Model file for the job. Use its own axes, mm. A direction names the side the tool comes from. Give positions to 0.01 mm unless a question says otherwise; leave off trailing zeros. Loops run counter-clockwise (first coordinate to the right, second up) from the corner with the lowest first, then second, coordinate; pieces in that order, holes last. Notation, with made-up numbers: (46, 87.5) - (86, 87.5) arc R11 ccw to (86, 101.5) - close; hole circle Ø6 at (-24, -26.75). An arc over 180 degrees is marked (long way). Use a Markdown table: item, result.
from build123d import *

# Parameters (mm, degrees)
EXTRUDE_1_DEPTH               = 3
SKETCH_2_W                    = 40
SKETCH_2_H                    = 29
EXTRUDE_2_DEPTH               = 4.3
EXTRUDE_3_DEPTH               = 3
SKETCH_4_W                    = 35.7
SKETCH_4_H                    = 29
EXTRUDE_4_DEPTH               = 4.3
SKETCH_5_W                    = 36
SKETCH_5_H                    = 8
CUT_EXTRUDE_1_DEPTH           = 2
CUT_EXTRUDE_1_DRAFT           = -30
CUT_EXTRUDE_1_PROFILE_2_DEPTH = 2
CUT_EXTRUDE_1_PROFILE_2_DRAFT = -30
SKETCH_5_W_2                  = 23.5
SKETCH_5_H_2                  = 8.8
CUT_EXTRUDE_1_PROFILE_3_DEPTH = 2
CUT_EXTRUDE_1_PROFILE_3_DRAFT = -30
SKETCH_6_W                    = 36
SKETCH_6_H                    = 8
CUT_EXTRUDE_2_DEPTH           = 2
CUT_EXTRUDE_2_DRAFT           = -30
CUT_EXTRUDE_2_PROFILE_2_DEPTH = 2
CUT_EXTRUDE_2_PROFILE_2_DRAFT = -30
SKETCH_6_W_2                  = 23.5
SKETCH_6_H_2                  = 8.8
CUT_EXTRUDE_2_PROFILE_3_DEPTH = 2
CUT_EXTRUDE_2_PROFILE_3_DRAFT = -30
EXTRUDE_START                 = -3
EXTRUDE_5_DEPTH               = 6
EXTRUDE_6_DEPTH               = 3
FILLET_2_R                    = 0.2


# Read off the part's stored shape, not the designer's step: the extrude step
with BuildPart() as part:
    # Sketch 1 → Extrude 1 (new body)
    with BuildSketch(Plane(origin=(0, 0, 0), x_dir=(1, 0, 0), z_dir=(0, 1, 0))):
        Polygon((0, 0), (0, 40), (-8, 40), (-8, 32), (-32, 8), (-40, 8), (-40, 0), align=None)
    extrude(amount=EXTRUDE_1_DEPTH)

    # Sketch 2 → Extrude 2 (add)
    with BuildSketch(Plane(origin=(0, 0, 0), x_dir=(0, 0, -1), z_dir=(1, 0, 0))):
        with Locations((20, 17.5)):
            Rectangle(SKETCH_2_W, SKETCH_2_H)
        with BuildLine():
            Line((27, 13.1), (15, 13.1))
            ThreePointArc((15, 13.1), (10.6, 17.5), (15, 21.9))
            Line((15, 21.9), (27, 21.9))
            ThreePointArc((27, 21.9), (31.4, 17.5), (27, 13.1))
        make_face(mode=Mode.SUBTRACT)
    extrude(amount=-EXTRUDE_2_DEPTH)

    # Sketch 3 → Extrude 3 (add)
    with BuildSketch(Plane(origin=(0, 32, 0), x_dir=(1, 0, 0), z_dir=(0, 1, 0))):
        Polygon((-4.3, 40), (0, 40), (0, 0), (-4.3, 0), (-40, 0), (-40, 8), (-32, 8), (-8, 32), (-8, 40), align=None)
    extrude(amount=EXTRUDE_3_DEPTH)

    # Sketch 4 → Extrude 4 (add)
    with BuildSketch(Plane.XY):
        with Locations((-22.15, 17.5)):
            Rectangle(SKETCH_4_W, SKETCH_4_H)
        with BuildLine():
            Line((-27, 21.9), (-15, 21.9))
            ThreePointArc((-15, 21.9), (-10.6, 17.5), (-15, 13.1))
            Line((-15, 13.1), (-27, 13.1))
            ThreePointArc((-27, 13.1), (-31.4, 17.5), (-27, 21.9))
        make_face(mode=Mode.SUBTRACT)
    extrude(amount=-EXTRUDE_4_DEPTH)


with BuildPart() as cut_extrude_1_tool:
    # Sketch 5 → Cut-Extrude 1 (with draft: the straight prism first)
    with BuildSketch(Plane(origin=(0, 0, 0), x_dir=(0, 0, -1), z_dir=(1, 0, 0))):
        with Locations((20, 28.5)):
            Rectangle(SKETCH_5_W, SKETCH_5_H)
    extrude(amount=-CUT_EXTRUDE_1_DEPTH)
    # Cut-Extrude 1: the draft: its side faces are tilted about the plane it starts from
    cut_extrude_1_sides = [cut_extrude_1_tool.faces().sort_by_distance(p)[0] for p in [
        (-1, 32.5, -20),
        (-1, 28.5, -2),
        (-1, 24.5, -20),
        (-1, 28.5, -38),
    ]]
    draft(cut_extrude_1_sides, Plane(origin=(0, 0, 0), x_dir=(0, 0, -1), z_dir=(1, 0, 0)), CUT_EXTRUDE_1_DRAFT)


with BuildPart() as part_1:
    add(part.part)

    # Cut-Extrude 1: cut by cut_extrude_1_tool
    add(cut_extrude_1_tool.part, mode=Mode.SUBTRACT)


with BuildPart() as cut_extrude_1_profile_2_tool:
    # Sketch 5 → Cut-Extrude 1 profile 2 (with draft: the straight prism first)
    with BuildSketch(Plane(origin=(0, 0, 0), x_dir=(0, 0, -1), z_dir=(1, 0, 0))):
        with Locations((20, 6.5)):
            Rectangle(SKETCH_5_W, SKETCH_5_H)
    extrude(amount=-CUT_EXTRUDE_1_PROFILE_2_DEPTH)
    # Cut-Extrude 1 profile 2: the draft: its side faces are tilted about the plane it starts from
    cut_extrude_1_profile_2_sides = [cut_extrude_1_profile_2_tool.faces().sort_by_distance(p)[0] for p in [
        (-1, 10.5, -20),
        (-1, 6.5, -2),
        (-1, 2.5, -20),
        (-1, 6.5, -38),
    ]]
    draft(cut_extrude_1_profile_2_sides, Plane(origin=(0, 0, 0), x_dir=(0, 0, -1), z_dir=(1, 0, 0)), CUT_EXTRUDE_1_PROFILE_2_DRAFT)


with BuildPart() as part_2:
    add(part_1.part)

    # Cut-Extrude 1 profile 2: cut by cut_extrude_1_profile_2_tool
    add(cut_extrude_1_profile_2_tool.part, mode=Mode.SUBTRACT)


with BuildPart() as cut_extrude_1_profile_3_tool:
    # Sketch 5 → Cut-Extrude 1 profile 3 (with draft: the straight prism first)
    with BuildSketch(Plane(origin=(0, 0, 0), x_dir=(0, 0, -1), z_dir=(1, 0, 0))):
        with Locations((19.75, 17.5)):
            Rectangle(SKETCH_5_W_2, SKETCH_5_H_2)
    extrude(amount=-CUT_EXTRUDE_1_PROFILE_3_DEPTH)
    # Cut-Extrude 1 profile 3: the draft: its side faces are tilted about the plane it starts from
    cut_extrude_1_profile_3_sides = [cut_extrude_1_profile_3_tool.faces().sort_by_distance(p)[0] for p in [
        (-1, 21.9, -19.75),
        (-1, 17.5, -8),
        (-1, 13.1, -19.75),
        (-1, 17.5, -31.5),
    ]]
    draft(cut_extrude_1_profile_3_sides, Plane(origin=(0, 0, 0), x_dir=(0, 0, -1), z_dir=(1, 0, 0)), CUT_EXTRUDE_1_PROFILE_3_DRAFT)


with BuildPart() as part_3:
    add(part_2.part)

    # Cut-Extrude 1 profile 3: cut by cut_extrude_1_profile_3_tool
    add(cut_extrude_1_profile_3_tool.part, mode=Mode.SUBTRACT)


with BuildPart() as cut_extrude_2_tool:
    # Sketch 6 → Cut-Extrude 2 (with draft: the straight prism first)
    with BuildSketch(Plane.XY):
        with Locations((-20, 6.5)):
            Rectangle(SKETCH_6_W, SKETCH_6_H)
    extrude(amount=-CUT_EXTRUDE_2_DEPTH)
    # Cut-Extrude 2: the draft: its side faces are tilted about the plane it starts from
    cut_extrude_2_sides = [cut_extrude_2_tool.faces().sort_by_distance(p)[0] for p in [
        (-20, 2.5, -1),
        (-2, 6.5, -1),
        (-20, 10.5, -1),
        (-38, 6.5, -1),
    ]]
    draft(cut_extrude_2_sides, Plane.XY, CUT_EXTRUDE_2_DRAFT)


with BuildPart() as part_4:
    add(part_3.part)

    # Cut-Extrude 2: cut by cut_extrude_2_tool
    add(cut_extrude_2_tool.part, mode=Mode.SUBTRACT)


with BuildPart() as cut_extrude_2_profile_2_tool:
    # Sketch 6 → Cut-Extrude 2 profile 2 (with draft: the straight prism first)
    with BuildSketch(Plane.XY):
        with Locations((-20, 28.5)):
            Rectangle(SKETCH_6_W, SKETCH_6_H)
    extrude(amount=-CUT_EXTRUDE_2_PROFILE_2_DEPTH)
    # Cut-Extrude 2 profile 2: the draft: its side faces are tilted about the plane it starts from
    cut_extrude_2_profile_2_sides = [cut_extrude_2_profile_2_tool.faces().sort_by_distance(p)[0] for p in [
        (-20, 24.5, -1),
        (-2, 28.5, -1),
        (-20, 32.5, -1),
        (-38, 28.5, -1),
    ]]
    draft(cut_extrude_2_profile_2_sides, Plane.XY, CUT_EXTRUDE_2_PROFILE_2_DRAFT)


with BuildPart() as part_5:
    add(part_4.part)

    # Cut-Extrude 2 profile 2: cut by cut_extrude_2_profile_2_tool
    add(cut_extrude_2_profile_2_tool.part, mode=Mode.SUBTRACT)


with BuildPart() as cut_extrude_2_profile_3_tool:
    # Sketch 6 → Cut-Extrude 2 profile 3 (with draft: the straight prism first)
    with BuildSketch(Plane.XY):
        with Locations((-19.75, 17.5)):
            Rectangle(SKETCH_6_W_2, SKETCH_6_H_2)
    extrude(amount=-CUT_EXTRUDE_2_PROFILE_3_DEPTH)
    # Cut-Extrude 2 profile 3: the draft: its side faces are tilted about the plane it starts from
    cut_extrude_2_profile_3_sides = [cut_extrude_2_profile_3_tool.faces().sort_by_distance(p)[0] for p in [
        (-19.75, 13.1, -1),
        (-8, 17.5, -1),
        (-19.75, 21.9, -1),
        (-31.5, 17.5, -1),
    ]]
    draft(cut_extrude_2_profile_3_sides, Plane.XY, CUT_EXTRUDE_2_PROFILE_3_DRAFT)


with BuildPart() as part_6:
    add(part_5.part)

    # Cut-Extrude 2 profile 3: cut by cut_extrude_2_profile_3_tool
    add(cut_extrude_2_profile_3_tool.part, mode=Mode.SUBTRACT)

    # Extrude 5 outline → Extrude 5 (add)
    with BuildSketch(Plane(origin=(0, 17.5, 0), x_dir=(1, 0, 0), z_dir=(0, 1, 0)).offset(EXTRUDE_START)):
        Polygon((0, 33.055050062), (0, 31.5), (3, 31.5), align=None)
        Polygon((0, 8), (3, 8), (-2, 10.591750104), (-2, 9.154700538), align=None)
    extrude(amount=EXTRUDE_5_DEPTH)

    # Sketch 8 → Extrude 6 (add, symmetric)
    with BuildSketch(Plane(origin=(0, 17.5, 0), x_dir=(1, 0, 0), z_dir=(0, 1, 0))):
        Polygon((-9.555050062, 0), (-8, -3), (-8, 0), align=None)
        Polygon((-34.091750104, 2), (-31.5, 2), (-31.5, -3), align=None)
        Polygon((-9.555050062, 0), (-8, 0), (-9.154700538, 2), (-10.591750104, 2), align=None)
    extrude(amount=EXTRUDE_6_DEPTH, both=True)

    # Fillet 2
    fillet_2_edges = [part_6.edges().sort_by_distance(p)[0] for p in [
        (3, 17.5, -8),
        (3, 17.5, -31.5),
        (-31.5, 17.5, 3),
        (-8, 17.5, 3),
    ]]
    fillet(fillet_2_edges, radius=FILLET_2_R)


solid = part_6.part
(1) Drill centre lines: probe 1 along Y at (x, z) = (-24, -4); probe 2 along Y at (x, z) = (-13.5, -5.5); probe 3 along Y at (x, z) = (-1, -36.5). Where is each one in solid material? Low to high. Write a range as [from, to].
Computed:
| item | result |
|---|---|
| probe 1 | [0, 13.1], [21.9, 35] |
| probe 2 | [0, 3], [32, 35] |
| probe 3 | [0, 3.08], [9.92, 25.08], [31.92, 35] |
(2) Mould opens along Z. For faces 1 (the flat face through (-29.78, 21.46, -0.76)), 2 (the flat face through (-31.5, 18, 1)), 3 (the flat face through (-0.99, 6.44, -37.43)) say: pulls with the +Z half, pulls with the -Z half, needs draft (parallel to the pull), parting line crosses it, or undercut.
Computed:
| item | result |
|---|---|
| face 1 | pulls with the +Z half |
| face 2 | needs draft |
| face 3 | undercut |
(3) Slice it at C-C, the plane y = 8. Write the cut outline in (x, z).
Computed:
| item | result |
|---|---|
| outline | (-40, -4.3) - (-4.3, -4.3) - (-4.3, -40) - (0, -40) - (0, -38) - (-2, -36.85) - (-2, -3.15) - (0, -2) - (0, 0) - (-2, 0) - (-3.15, -2) - (-36.85, -2) - (-38, 0) - (-40, 0) - close |
(4) Slice it at D-D, the plane y = 18. Count the separate pieces of the cut face and the enclosed holes in it, plus the area to 3 significant figures.
Computed:
| item | result |
|---|---|
| separate pieces | 3 |
| enclosed holes | 0 |
| area | 154 mm² |
(5) Slice it at B-B, the plane z = -19. Write the cut outline in (x, y).
Computed:
| item | result |
|---|---|
| outline | (-21, 0) - (0, 0) - (0, 2.5) - (-2, 3.65) - (-2, 9.35) - (0, 10.5) - (0, 13.1) - (-4.3, 13.1) - (-4.3, 3) - (-21, 3) - close; (-21, 32) - (-4.3, 32) - (-4.3, 21.9) - (0, 21.9) - (0, 24.5) - (-2, 25.65) - (-2, 31.35) - (0, 32.5) - (0, 35) - (-21, 35) - close |
(6) 3-axis set-ups, long thin cutter, end or side, ignore diameter. For faces 4 (the flat face through (-20.25, 9.93, -0.99)), 5 (the flat face through (-14, 3, -14)), 6 (the flat face through (0, 14.5, -9)): which of +Z, -Z, +X, -X, +Y, -Y reach the whole face in a straight line?
Computed:
| item | result |
|---|---|
| face 4 | +Z |
| face 5 | -Z, -X |
| face 6 | +X |
(7) Pin check, flat tips, straight feed: P1, Ø4, axis at x = -11, y = 21, coming from the -Z side; P2, Ø1.7, axis at x = -32, z = 1.5, coming from the -Y side; P3, Ø6, axis at x = -4.5, y = 31, coming from the +Z side. Stop position of each tip, or through.
Computed:
| item | result |
|---|---|
| P1 | z = -4.3 |
| P2 | y = 14.5 |
| P3 | z = 0 |
(8) Slice it at A-A, the plane x = -21. Write the cut outline in (y, z), plus the area to 3 significant figures.
Computed:
| item | result |
|---|---|
| outline | (0, -19) - (3, -19) - (3, -4.3) - (13.1, -4.3) - (13.1, 0) - (10.5, 0) - (9.35, -2) - (3.65, -2) - (2.5, 0) - (0, 0) - close; (21.9, -4.3) - (32, -4.3) - (32, -19) - (35, -19) - (35, 0) - (32.5, 0) - (31.35, -2) - (25.65, -2) - (24.5, 0) - (21.9, 0) - close |
| area | 173 mm² |
